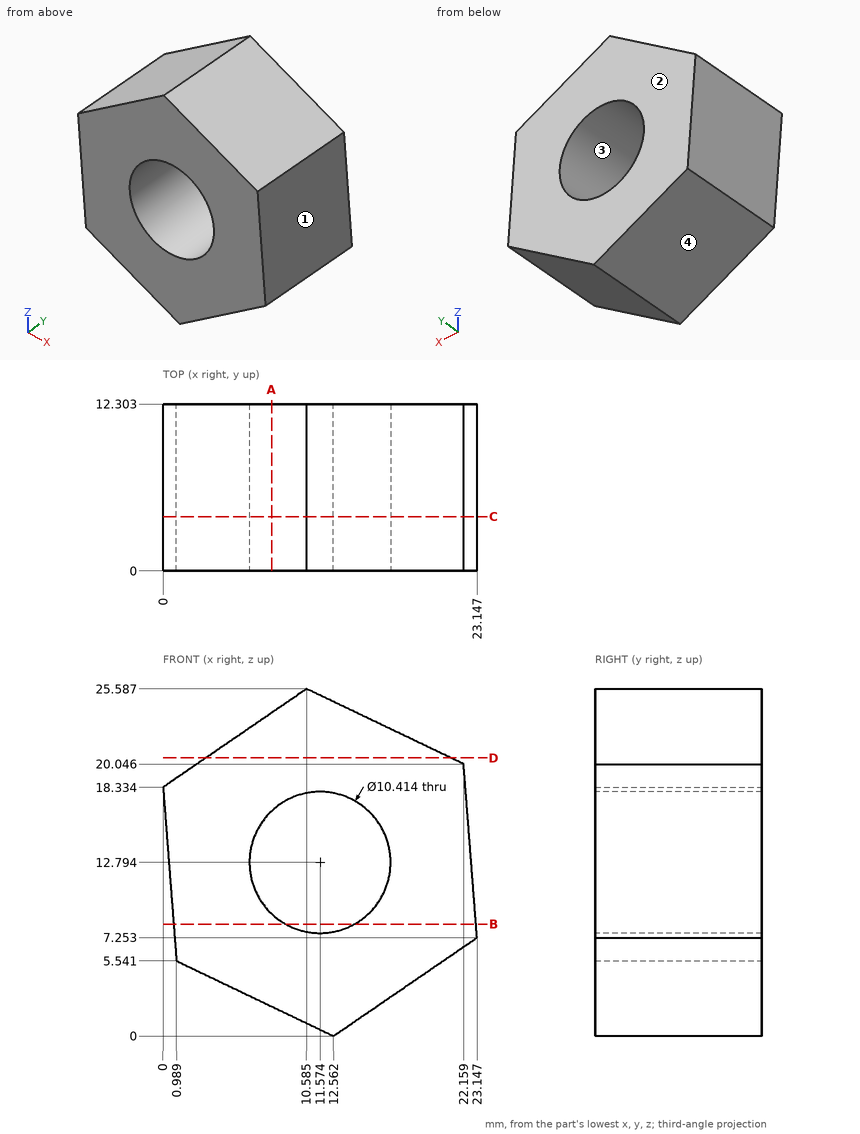
Geometry check sheet. Reference: drawing and pictorial views, mm from the part's lowest x, y, z. Give positions to 0.01 mm unless a question says otherwise; leave off trailing zeros. Loops run counter-clockwise (first coordinate to the right, second up) from the corner with the lowest first, then second, coordinate; pieces in that order, holes last. Notation, with made-up numbers: (-38, -8) -> (-3, -8) arc R19 ccw to (-3, 29) -> close; hole circle Ø1 at (32.5, 12.25). An arc over 180 degrees is marked (long way). Answer in a Markdown table with one row per item. Add a question column.
1) Cross-section at A-A on x = 8. Record the boundary of the cut face in (y, z) (1 decimal).
2) Gauge pin test, flat ends, axial feed: P1, Ø3, axis at x = 6, y = 8, coming from the +Z side; P2, Ø3, axis at x = 20.5, y = 6, coming from the -Z side; P3, Ø2, axis at x = 7.5, y = 3.5, coming from the +Z side. Record the tip position at first contact, or that the pin passes through.
3) Cross-section at B-B on z = 8.25. Record the boundary of the cut face in (x, y), and give its area (3 significant figures).
4) Cross-section at C-C on y = 4. Record the boundary of the cut face in (x, z) (1 decimal).
5) Material ranges on probe 1 along X at (y, z) = (11, 8.75) (1 decimal); probe 2 along Z at (x, y) = (13, 4.75) (1 decimal); probe 3 along X at (y, z) = (5.25, 16) (1 decimal), recorded low to high. Write a range as from..to.
6) Cross-section at D-D on z = 20.5. Record the boundary of the cut face in (x, y).
7) Draft check along Z on the marked faces 1, 2, 3 and 4. Enter one of: pulls with the +Z half, pulls with the -Z half, needs draft (parallel to the pull), parting line crosses it, or undercut.
Outcome:
| question | item | result |
|---|---|---|
| 1 | outline | (0, 2.2) -> (12.3, 2.2) -> (12.3, 9) -> (0, 9) -> close; (0, 16.6) -> (12.3, 16.6) -> (12.3, 23.8) -> (0, 23.8) -> close |
| 2 | P1 | stops at z = 23.47 |
| 2 | P2 | stops at z = 4.41 |
| 2 | P3 | stops at z = 24.16 |
| 3 | outline | (0.78, 0) -> (9.03, 0) -> (9.03, 12.3) -> (0.78, 12.3) -> close; (14.12, 0) -> (23.07, 0) -> (23.07, 12.3) -> (14.12, 12.3) -> close |
| 3 | area | 212 mm^2 |
| 4 | outline | (0, 18.3) -> (1, 5.5) -> (12.6, 0) -> (23.1, 7.3) -> (22.2, 20) -> (10.6, 25.6) -> close; hole circle Ø10.4 at (11.6, 12.8) |
| 5 | probe 1 | x = 0.7..8.3, 14.9..23 |
| 5 | probe 2 | z = 0.3..7.8, 17.8..24.4 |
| 5 | probe 3 | x = 0.2..7.5, 15.7..22.5 |
| 6 | outline | (3.16, 0) -> (21.21, 0) -> (21.21, 12.3) -> (3.16, 12.3) -> close |
| 7 | face 1 | pulls with the +Z half |
| 7 | face 2 | needs draft |
| 7 | face 3 | undercut |
| 7 | face 4 | pulls with the -Z half |
